Geometry: see drawing. Coordinates: mm, zero at the bounding-box minimum. A direction names the side the tool comes from. Round coordinates to 2 decimals unless told otherwise and drop trailing zeros. Write each loop counter-clockwise with the first axis right and the second up, starting at its lowest first coordinate (ties: lowest second). Pieces come first, ordered by that corner, then holes. Notation, with made-up numbers: M -21.75,42 L 20.25,42 A18 ccw 20.25,68 Z; hole C 70.5,-36 d8. An arc over 180 degrees is marked long. Use a Markdown table: item, result.
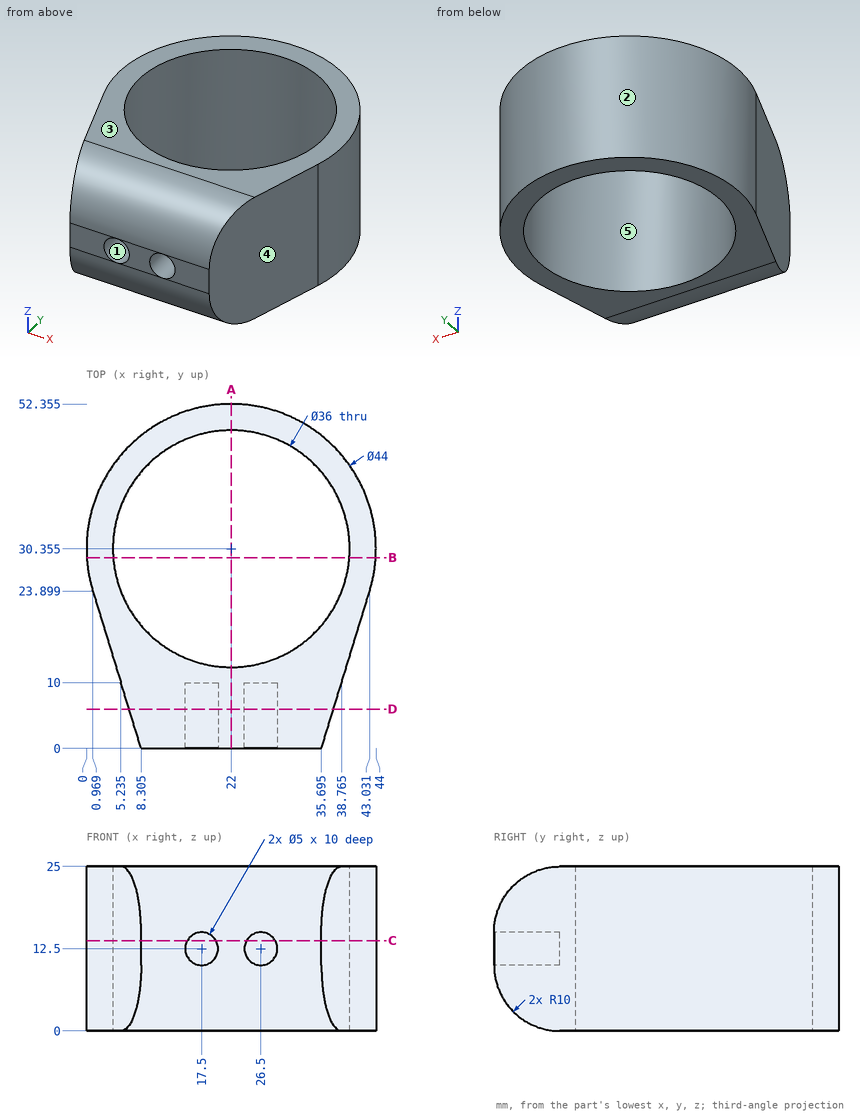
Q1. Section B-B on y = 29. Return loops of the section in (x, z).
Results are:
| item | result |
|---|---|
| outline | M 0.04,0 L 4.05,0 L 4.05,25 L 0.04,25 Z; M 39.95,0 L 43.96,0 L 43.96,25 L 39.95,25 Z |
Q2. Section A-A on x = 22. Return loops of the section in (y, z) (1 decimal).
Results are:
| item | result |
|---|---|
| outline | M 0,10 A10 ccw 10,0 L 12.4,0 L 12.4,25 L 10,25 A10 ccw 0,15 Z; M 48.4,0 L 52.4,0 L 52.4,25 L 48.4,25 Z |
Q3. Reachability of the marked faces 1 and 2 from +Z, -Z, +X, -X, +Y, -Y: full face, straight path, thin tool, end or side. Return the list, or none.
Results are:
| item | result |
|---|---|
| face 1 | -Y |
| face 2 | +Z, -Z |
Q4. First-contact query: pin 1 Ø8 at (x, z) = (17.5, 12.5) entering from +Y; pin 2 Ø3 at (x, z) = (26.5, 12.5) entering from +Y; pin 3 Ø8 at (y, z) = (7.5, 16.5) entering from -X (1 decimal). Flat tips, straight axial feed; report the tip coordinate or a pass-through.
Results are:
| item | result |
|---|---|
| pin 1 | y = 52.35 |
| pin 2 | y = 52.15 |
| pin 3 | x = 4.8 |
Q5. Mould query, pull axis X, two halves, no side actions, for the marked faces 3, 4 and 5. Classes: +X half, -X half, draft (parallel to the pull), parting line (faces both ways), or undercut.
Results are:
| item | result |
|---|---|
| face 3 | draft |
| face 4 | +X half |
| face 5 | undercut |
Q6. Line query: L1, parallel to X at y = 6, z = 12.25; L2, parallel to Y at x = 21, z = 14.75; L3, parallel to X at y = 35.5, z = 2.5. Output: solid intervals per line, ascending.
Results are:
| item | result |
|---|---|
| L1 | 6.46 to 15.01, 19.99 to 24.01, 28.99 to 37.54 |
| L2 | 0 to 12.38, 48.33 to 52.33 |
| L3 | 0.61 to 4.75, 39.25 to 43.39 |
Q7. Section C-C on z = 13.75. Return loops of the section in (x, y) (1 decimal).
Results are:
| item | result |
|---|---|
| outline | M 1,23.9 L 8.3,0 L 15.3,0 L 15.3,10 L 19.7,10 L 19.7,0 L 24.3,0 L 24.3,10 L 28.7,10 L 28.7,0 L 35.7,0 L 43,23.9 A22 ccw long Z; hole C 22,30.4 d36 |
Q8. Section D-D on y = 6. Return loops of the section in (x, z) (1 decimal), plus the area to 3 significant figures.
Results are:
| item | result |
|---|---|
| outline | M 6.5,0.8 L 37.5,0.8 L 37.5,24.2 L 6.5,24.2 Z; hole C 17.5,12.5 d5; hole C 26.5,12.5 d5 |
| area | 686 mm^2 |
